Verification items for the finished model (mm, model axes). A direction names the side the tool comes from. Round coordinates to 2 decimals unless told otherwise and drop trailing zeros. Write each loop counter-clockwise with the first axis right and the second up, starting at its lowest first coordinate (ties: lowest second). Pieces come first, ordered by that corner, then holes. Notation, with made-up numbers: M 47,26 L 105,26 A19 cw 105,42 Z; hole C -15.75,44 d10. An arc over 180 degrees is marked long. Answer in a Markdown table with one row per item. Add a question column.
1. Go/stop test with flat-tipped pins: pin 1 Ø5 at (x, z) = (15.5, 13.5) entering from +Y; pin 2 Ø8 at (x, y) = (-12.5, 82) entering from +Z; pin 3 Ø3 at (x, y) = (-12, 30.5) entering from -Z. Record where each tip stops, or that it passes through.
2. Draft check along Y on faces 1 (the flat face through (18, 20, -3)), 2 (the flat face through (0, 20, 0)), 3 (the cylindrical face through (7.509, 9.86, 23.846)). Enter one of: pulls with the +Y half, pulls with the -Y half, needs draft (parallel to the pull), parting line crosses it, or undercut.
3. Sectioned sample at A-A on x = 20.5. Record the cut outline in (y, z).
4. Material ranges on probe 1 along Y at (x, z) = (4.5, 0.5); probe 2 along X at (y, z) = (66.5, 5.5); probe 3 along X at (y, z) = (34, -10), recorded low to high.
5. Set-up check for faces 4 (the conical face through (11.033, 60.56, -3.474)), 5 (the flat face through (0, 0, 0)): record each of +Z, -Z, +X, -X, +Y, -Y from which the full face is reachable in a straight line by a thin tool's end or side.
```python
from build123d import *

# Parameters (mm, degrees)
CROQUIS1_R              = 25
SALIENTE_EXTRUIR1_DEPTH = 20
CROQUIS5_R              = 9.5
CORTAR_EXTRUIR1_DEPTH   = 80
CORTAR_EXTRUIR1_DRAFT   = 3


with BuildPart() as part:
    # Croquis1 → Saliente-Extruir1 (new body)
    with BuildSketch(Plane(origin=(0, 0, 0), x_dir=(1, 0, 0), z_dir=(0, 1, 0))):
        with Locations(Location((0, 0, 0), (0, 0, 270))):
            Circle(CROQUIS1_R)
    extrude(amount=SALIENTE_EXTRUIR1_DEPTH)

    # Recubrir1: read off the stored shape, not the designer's step
    # Recubrir1: loft between two sections, ruled curve by curve
    recubrir1_from = [
        Edge.make_bspline([(-9.844568518, 20, 15.069322171), (20.294075824, 20, 34.758459207), (39.98321286, 20, 4.619814865), (9.844568518, 20, -15.069322171), (-20.294075824, 20, -34.758459207), (-39.98321286, 20, -4.619814865), (-9.844568518, 20, 15.069322171)], [0, 0, 0, 0, 0.5, 0.5, 0.5, 1, 1, 1, 1], 3, [1, 0.333333333, 0.333333333, 1, 0.333333333, 0.333333333, 1]),
    ]
    recubrir1_to = [
        Edge.make_bspline([(2.388538874, 100, 12.269673266), (26.927885406, 100, 7.492595517), (22.150807657, 100, -17.046751015), (-2.388538874, 100, -12.269673266), (-26.927885406, 100, -7.492595517), (-22.150807657, 100, 17.046751015), (2.388538874, 100, 12.269673266)], [0, 0, 0, 0, 0.5, 0.5, 0.5, 1, 1, 1, 1], 3, [1, 0.333333333, 0.333333333, 1, 0.333333333, 0.333333333, 1]),
    ]
    recubrir1 = Solid(Shell([*[Face.make_surface_from_curves(recubrir1_from[k], recubrir1_to[k]) for k in range(1)], Face(Wire(recubrir1_from)), Face(Wire(recubrir1_to))]))
    add(recubrir1)


with BuildPart() as cortar_extruir1_tool:
    # Croquis5 → Cortar-Extruir1 (with draft: the straight prism first)
    with BuildSketch(Plane(origin=(0, 100, 0), x_dir=(1, 0, 0), z_dir=(0, 1, 0))):
        Circle(CROQUIS5_R)
    extrude(amount=-CORTAR_EXTRUIR1_DEPTH)
    # Cortar-Extruir1: the draft: its side faces are tilted about the plane it starts from
    cortar_extruir1_sides = [cortar_extruir1_tool.faces().sort_by_distance(p)[0] for p in [
        (-9.5, 60, 0),
    ]]
    draft(cortar_extruir1_sides, Plane(origin=(0, 100, 0), x_dir=(1, 0, 0), z_dir=(0, 1, 0)), CORTAR_EXTRUIR1_DRAFT)


with BuildPart() as part_1:
    add(part.part)

    # Cortar-Extruir1: cut by cortar_extruir1_tool
    add(cortar_extruir1_tool.part, mode=Mode.SUBTRACT)


solid = part_1.part
```
Geometry check:
| question | item | result |
|---|---|---|
| 1 | pin 1 | stops at y = 20 |
| 1 | pin 2 | stops at z = 9.72 |
| 1 | pin 3 | stops at z = -13.2 |
| 2 | face 1 | pulls with the +Y half |
| 2 | face 2 | undercut |
| 2 | face 3 | needs draft |
| 3 | outline | M 0,-14.31 L 20,-14.31 L 20,14.31 L 0,14.31 Z |
| 4 | probe 1 | y = 0 to 20 |
| 4 | probe 2 | x = -12.57 to -9.82, 9.82 to 12.57 |
| 4 | probe 3 | x = -13.11 to -8.24, 8.24 to 13.11 |
| 5 | face 4 | none |
| 5 | face 5 | +Z, -Z, +X, -X, -Y |
